from build123d import *

# Parameters (mm, degrees)
IZIM1_W                     = 15
IZIM1_H                     = 19
Y_KSEKLIK_EKSTR_ZYON1_DEPTH = 16
RADYUS1_R                   = 0.1
IZIM2_R                     = 0.25
Y_KSEKLIK_EKSTR_ZYON2_DEPTH = 2


with BuildPart() as part:
    # Çizim1 → Yükseklik-Ekstrüzyon1 (new body)
    with BuildSketch(Plane(origin=(0, 0, 0), x_dir=(1, 0, 0), z_dir=(0, 1, 0))):
        Rectangle(IZIM1_W, IZIM1_H)
    extrude(amount=Y_KSEKLIK_EKSTR_ZYON1_DEPTH)

    # Radyus1
    radyus1_edges = [part.edges().sort_by_distance(p)[0] for p in [
        (-7.5, 16, 0),
        (0, 16, 9.5),
        (7.5, 16, 0),
        (0, 16, -9.5),
        (7.5, 8, 9.5),
        (-7.5, 8, 9.5),
        (-7.5, 8, -9.5),
        (7.5, 8, -9.5),
    ]]
    fillet(radyus1_edges, radius=RADYUS1_R)

    # Çizim2 → Yükseklik-Ekstrüzyon2 (add)
    with BuildSketch(Plane.XZ):
        with Locations((6, 6.25)):
            Circle(IZIM2_R)
        with Locations((-6, 6.25)):
            Circle(IZIM2_R)
        with Locations((6, -6.25)):
            Circle(IZIM2_R)
        with Locations((-6, -6.25)):
            Circle(IZIM2_R)
        with Locations((0, -8.25)):
            Circle(IZIM2_R)
    extrude(amount=Y_KSEKLIK_EKSTR_ZYON2_DEPTH)

    # Çizim3 → Döndür1 (revolve)
    with BuildSketch(Plane.ZY.offset(6)):
        with BuildLine():
            Line((-6.25, -2), (-6.25, -1))
            Line((-6.25, -1), (-5.25, -1))
            add(Edge.make_bspline(
                [(-6.25, -2), (-5.440038175, -1.628390392), (-5.25, -1)],
                knots=[0, 0, 0, 0.619923651, 0.619923651, 0.619923651], degree=2))
        make_face()
    revolve(axis=Axis((-6, -2, -6.25), (0, 1, 0)))

    # Çizim4 → Döndür2 (revolve)
    with BuildSketch(Plane.ZY.offset(6)):
        with BuildLine():
            Line((6.25, -2), (6.25, -1))
            Line((6.25, -1), (7.25, -1))
            add(Edge.make_bspline(
                [(6.25, -2), (7.064808885, -1.63039811), (7.25, -1)],
                knots=[0, 0, 0, 0.629617769, 0.629617769, 0.629617769], degree=2))
        make_face()
    revolve(axis=Axis((-6, -2, 6.25), (0, 1, 0)))

    # Çizim5 → Döndür3 (revolve)
    with BuildSketch(Plane(origin=(6, 0, 0), x_dir=(0, 0, -1), z_dir=(1, 0, 0))):
        with BuildLine():
            Line((-6.25, -2), (-6.25, -1))
            Line((-6.25, -1), (-7.25, -1))
            add(Edge.make_bspline(
                [(-6.25, -2), (-7.108302041, -1.648413565), (-7.25, -1)],
                knots=[0, 0, 0, 0.716604082, 0.716604082, 0.716604082], degree=2))
        make_face()
    revolve(axis=Axis((6, -2, 6.25), (0, 1, 0)))

    # Çizim6 → Döndür4 (revolve)
    with BuildSketch(Plane(origin=(6, 0, 0), x_dir=(0, 0, -1), z_dir=(1, 0, 0))):
        with BuildLine():
            Line((6.25, -2), (6.25, -1))
            Line((6.25, -1), (7.25, -1))
            add(Edge.make_bspline(
                [(6.25, -2), (7.16916064, -1.673622022), (7.25, -1)],
                knots=[0, 0, 0, 0.838321281, 0.838321281, 0.838321281], degree=2))
        make_face()
    revolve(axis=Axis((6, -2, -6.25), (0, 1, 0)))

    # Çizim7 → Döndür5 (revolve)
    with BuildSketch(Plane(origin=(0, 0, 0), x_dir=(0, 0, -1), z_dir=(1, 0, 0))):
        with BuildLine():
            Line((8.25, -2), (8.25, -1))
            Line((8.25, -1), (9.25, -1))
            add(Edge.make_bspline(
                [(9.25, -1), (8.854156938, -1.651239765), (8.25, -2)],
                knots=[0, 0, 0, 0.716230024, 0.716230024, 0.716230024], degree=2))
        make_face()
    revolve(axis=Axis((0, -2, -8.25), (0, 1, 0)))


solid = part.part
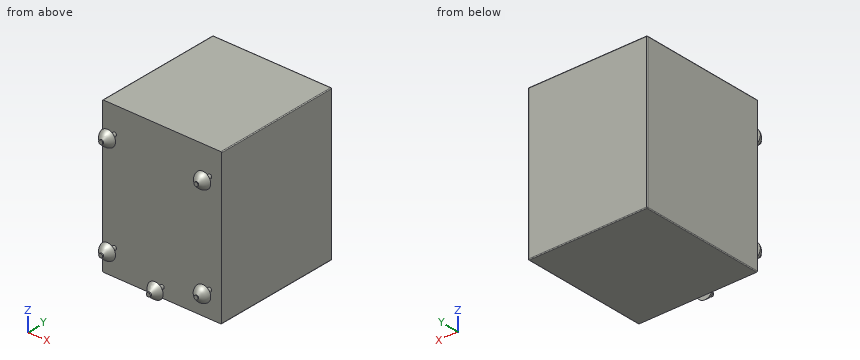
Verification items for the finished model (mm, model axes). Coordinates: 2 decimals unless noted, no trailing zeros. Write each loop counter-clockwise with the first axis right and the second up, starting at its lowest first coordinate (ties: lowest second). Pieces come first, ordered by that corner, then holes. Notation, with made-up numbers: M 50,-30.5 L 92,-30.5 A12 ccw 92,-13.5 Z; hole C -40,-37.75 d7. An arc over 180 degrees is marked long. Use CSV: the item, a comma, the result in double quotes.
Q1. Section check B-B, the plane x = -3. Enter the section's corners in (y, z), and give its area (3 significant figures).
Computed values:
outline,"M 0,-9.5 L 15.9,-9.5 A0.1 ccw 16,-9.4 L 16,9.4 A0.1 ccw 15.9,9.5 L 0,9.5 Z"
area,"304 mm²"
Q2. Thickness scan on line 1 along Y through (x, z) = (5, 1). Record the ranges inside material, lowest first. Write a range as [from, to].
Computed values:
line 1,"[0, 16]"
Q3. Section check A-A, the plane y = -0.25. Enter the section's corners in (x, z), and give its area (3 significant figures).
Computed values:
outline,"C -6,-6.25 d0.5; C -6,6.25 d0.5; C 0,-8.25 d0.5; C 6,-6.25 d0.5; C 6,6.25 d0.5"
area,"0.982 mm²"
Q4. Section check C-C, the plane z = 7. State how many separate pieces and enclosed holes the cut face has, and give its area (3 significant figures).
Computed values:
separate pieces,"3"
enclosed holes,"0"
area,"241 mm²"
Q5. Section check D-D, the plane z = 2.5. Enter the section's corners in (x, y), and give its area (3 significant figures).
Computed values:
outline,"M -7.5,0 L 7.5,0 L 7.5,15.9 A0.1 ccw 7.4,16 L -7.4,16 A0.1 ccw -7.5,15.9 Z"
area,"240 mm²"
